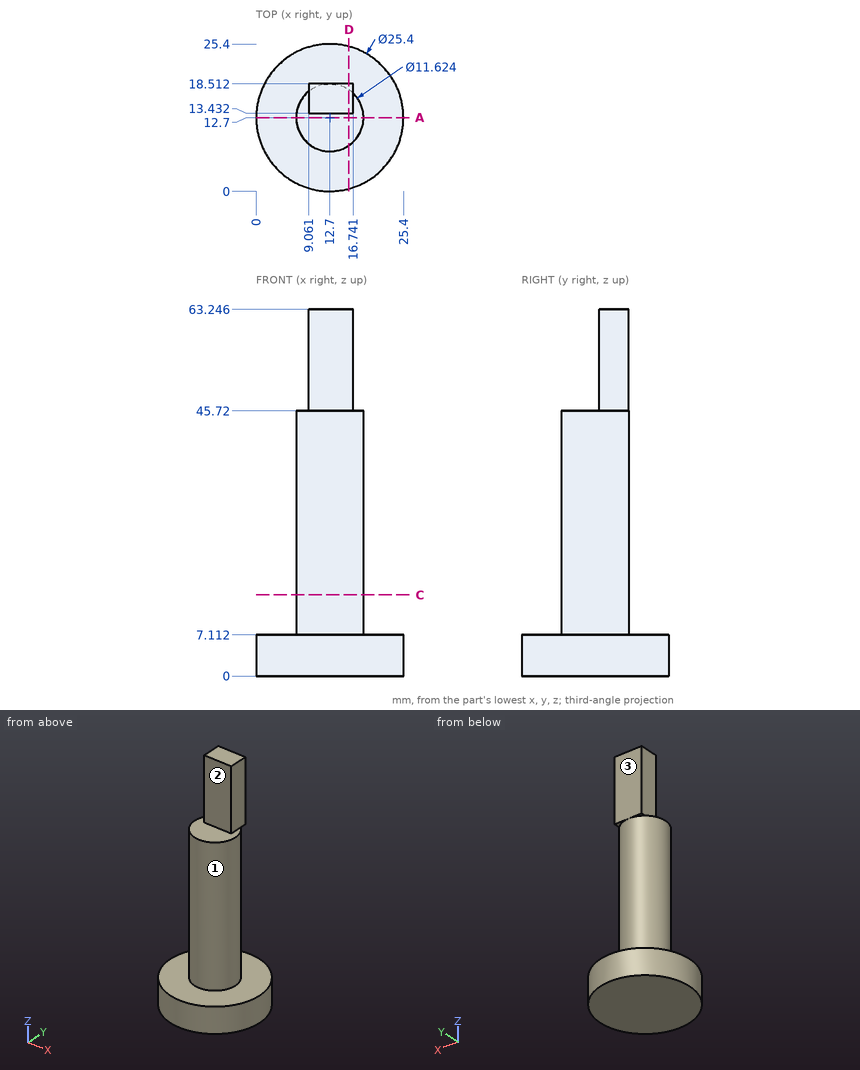
Job drawing, mm, ordinate dimensions from the low corner. One solid piece. A direction names the side the tool comes from. Round coordinates to 2 decimals unless told otherwise and drop trailing zeros. Loops run counter-clockwise (first coordinate to the right, second up) from the corner with the lowest first, then second, coordinate; pieces in that order, holes last.
Item 1: 3-axis set-ups, long thin cutter, end or side, ignore diameter. For the marked faces 1, 2 and 3: which of +Z, -Z, +X, -X, +Y, -Y reach the whole face in a straight line?
Item 2: Drill centre lines: line 1 (Z direction, x = 15, y = 24); line 2 (X direction, y = 13.75, z = 56); line 3 (Z direction, x = 18, y = 12). Where is each one in solid material? Low to high.
Item 3: Cut at D-D, the plane x = 16. Give the cut face in (y, z), then the cut area to 3 significant figures.
Item 4: Cut at A-A, the plane y = 12.7. Give the cut face in (x, z).
Item 5: Cut at C-C, the plane z = 14. Give the cut face in (x, y).
Item 6: Drop flat-ended pins along their axis: P1, Ø4, axis at x = 12.5, z = 51.5, coming from the -Y side; P2, Ø6, axis at x = 4, y = 17.5, coming from the -Z side; P3, Ø3, axis at y = 18, z = 34.5, coming from the -X side; P4, Ø5, axis at x = 13.5, z = 10.5, coming from the +Y side. Give the stop position or say it passes through.
A:
1. face 1: none
1. face 2: +Z, +X, -X, -Y
1. face 3: +Z, +X, -X, +Y
2. line 1: z = 0 to 7.11
2. line 2: x = 9.06 to 16.74
2. line 3: z = 0 to 45.72
3. outline: (0.44, 0) - (24.96, 0) - (24.96, 7.11) - (17.48, 7.11) - (17.48, 45.72) - (18.51, 45.72) - (18.51, 63.25) - (13.43, 63.25) - (13.43, 45.72) - (7.92, 45.72) - (7.92, 7.11) - (0.44, 7.11) - close
3. area: 633 mm2
4. outline: (0, 0) - (25.4, 0) - (25.4, 7.11) - (18.51, 7.11) - (18.51, 45.72) - (6.89, 45.72) - (6.89, 7.11) - (0, 7.11) - close
5. outline: circle Ø11.62 at (12.7, 12.7)
6. P1: stops at y = 13.43
6. P2: stops at z = 0
6. P3: stops at x = 8.3
6. P4: stops at y = 18.51
